from build123d import *

# Parameters (mm, degrees)
F0_R     = 14.2875
F1_DEPTH = 25.4
F2_DEPTH = 50.8


with BuildPart() as f1:
    # F0 (on Top) → F1 (new body)
    with BuildSketch(Plane.XY):
        with BuildLine():
            Line((9.780704698, 26.8489932886), (0, 28.575))
            ThreePointArc((0, 28.575), (-28.575, 0), (0, -28.575))
            Line((0, -28.575), (9.780704698, -26.8489932886))
            ThreePointArc((9.780704698, -26.8489932886), (23.4095521288, -16.3866864902), (28.575, 0))
            ThreePointArc((28.575, 0), (23.4095521288, 16.3866864902), (9.780704698, 26.8489932886))
        make_face()
        with BuildLine():
            ThreePointArc((-13.4703841816, 4.7625), (0, 14.2875), (13.4703841816, 4.7625))
            Line((13.4703841816, 4.7625), (19.05, 4.7625))
            Line((19.05, 4.7625), (19.05, -4.7625))
            Line((19.05, -4.7625), (13.4703841816, -4.7625))
            ThreePointArc((13.4703841816, -4.7625), (0, -14.2875), (-13.4703841816, -4.7625))
            Line((-13.4703841816, -4.7625), (-19.05, -4.7625))
            Line((-19.05, -4.7625), (-19.05, 4.7625))
            Line((-19.05, 4.7625), (-13.4703841816, 4.7625))
        make_face(mode=Mode.SUBTRACT)
        with BuildLine():
            ThreePointArc((9.780704698, 26.8489932886), (4.9659159165, 28.1401901932), (0, 28.575))
            Line((0, 28.575), (9.780704698, 26.8489932886))
        make_face()
        with BuildLine():
            Line((53.975, 19.05), (9.780704698, 26.8489932886))
            ThreePointArc((9.780704698, 26.8489932886), (23.4095521288, 16.3866864902), (28.575, 0))
            ThreePointArc((28.575, 0), (23.4095521288, -16.3866864902), (9.780704698, -26.8489932886))
            Line((9.780704698, -26.8489932886), (53.975, -19.05))
            ThreePointArc((53.975, -19.05), (34.925, 0), (53.975, 19.05))
        make_face()
        with BuildLine():
            ThreePointArc((73.025, 0), (67.4453841816, 13.4703841816), (53.975, 19.05))
            ThreePointArc((53.975, 19.05), (34.925, 0), (53.975, -19.05))
            ThreePointArc((53.975, -19.05), (67.4453841816, -13.4703841816), (73.025, 0))
        make_face()
        with Locations((53.975, 0)):
            Circle(F0_R, mode=Mode.SUBTRACT)
        with BuildLine():
            ThreePointArc((-13.4703841816, -4.7625), (-14.2875, 0), (-13.4703841816, 4.7625))
            Line((-13.4703841816, 4.7625), (-19.05, 4.7625))
            Line((-19.05, 4.7625), (-19.05, -4.7625))
            Line((-19.05, -4.7625), (-13.4703841816, -4.7625))
        make_face()
    extrude(amount=F1_DEPTH)

    # F0 (on Top) → F2 (join)
    with BuildSketch(Plane.XY):
        with BuildLine():
            ThreePointArc((9.780704698, 26.8489932886), (4.9659159165, 28.1401901932), (0, 28.575))
            Line((0, 28.575), (9.780704698, 26.8489932886))
        make_face()
        with BuildLine():
            Line((9.780704698, -26.8489932886), (0, -28.575))
            ThreePointArc((0, -28.575), (4.9659159165, -28.1401901932), (9.780704698, -26.8489932886))
        make_face()
        with BuildLine():
            Line((9.780704698, 26.8489932886), (0, 28.575))
            ThreePointArc((0, 28.575), (-28.575, 0), (0, -28.575))
            Line((0, -28.575), (9.780704698, -26.8489932886))
            ThreePointArc((9.780704698, -26.8489932886), (23.4095521288, -16.3866864902), (28.575, 0))
            ThreePointArc((28.575, 0), (23.4095521288, 16.3866864902), (9.780704698, 26.8489932886))
        make_face()
        with BuildLine():
            ThreePointArc((-13.4703841816, 4.7625), (0, 14.2875), (13.4703841816, 4.7625))
            Line((13.4703841816, 4.7625), (19.05, 4.7625))
            Line((19.05, 4.7625), (19.05, -4.7625))
            Line((19.05, -4.7625), (13.4703841816, -4.7625))
            ThreePointArc((13.4703841816, -4.7625), (0, -14.2875), (-13.4703841816, -4.7625))
            Line((-13.4703841816, -4.7625), (-19.05, -4.7625))
            Line((-19.05, -4.7625), (-19.05, 4.7625))
            Line((-19.05, 4.7625), (-13.4703841816, 4.7625))
        make_face(mode=Mode.SUBTRACT)
        with BuildLine():
            ThreePointArc((-13.4703841816, -4.7625), (-14.2875, 0), (-13.4703841816, 4.7625))
            Line((-13.4703841816, 4.7625), (-19.05, 4.7625))
            Line((-19.05, 4.7625), (-19.05, -4.7625))
            Line((-19.05, -4.7625), (-13.4703841816, -4.7625))
        make_face()
    extrude(amount=F2_DEPTH)


solid = f1.part
Geometry check sheet. Reference: the model listing, model coordinates, mm. A direction names the side the tool comes from. Round coordinates to 2 decimals unless told otherwise and drop trailing zeros. Write each loop counter-clockwise with the first axis right and the second up, starting at its lowest first coordinate (ties: lowest second). Pieces come first, ordered by that corner, then holes. Notation, with made-up numbers: (28, 63) -> (75, 63) arc R15 cw to (75, 68) -> close; hole circle Ø9 at (65, -28). An arc over 180 degrees is marked (long way). One line per item, written item: value. Start each with the question number.
(1) Cross-section at A-A, the plane x = 0. Record the cut outline in (y, z) (1 decimal), and give its area (3 significant figures).
(2) Go/stop test with flat-tipped pins: pin 1 Ø2 at (x, y) = (45.5, 12.5) entering from +Z; pin 2 Ø6 at (y, z) = (-2.5, 12) entering from -X (3 decimals); pin 3 Ø1.7 at (x, z) = (17, 17.5) entering from -Y (3 decimals); pin 4 Ø3 at (x, y) = (13, -8) entering from -Z. Record where each tip stops, or that it passes through.
(3) Cross-section at B-B, the plane z = 13. Give the number of separate pieces and of enclosed holes in the cut face, and give its area (3 significant figures).
(4) Access from +Z, -Z, +X, -X, +Y, -Y to the whole of each face (thin tool, end or side, straight path). Record for faces 4 (the cylindrical face through (-27.895, 6.194, 25.044)), 5 (the flat face through (22, 0, 0)), 6 (the flat face through (16, -4.762, 25)).
(5) Cross-section at D-D, the plane x = 66. Record the cut outline in (y, z).
(6) Draft check along Y on faces 1 (the flat face through (19.05, 0, 25)), 2 (the cylindrical face through (73.02, -0.42, 12.52)), 3 (the flat face through (31.6, -23, 12.5)). Enter one of: +Y half, -Y half, draft (parallel to the pull), parting line (faces both ways), or undercut.
(7) Scan lines: line 1 (X direction, y = -0.5, z = 38); line 2 (Z direction, x = 37, y = 16.5); line 3 (Y direction, x = -6, z = 34). Record each from-to range of solid material in increasing order. Write a range as [from, to].
Answer:
1. outline: (-28.6, 0) -> (-14.3, 0) -> (-14.3, 50.8) -> (-28.6, 50.8) -> close; (14.3, 0) -> (28.6, 0) -> (28.6, 50.8) -> (14.3, 50.8) -> close
1. area: 1,450 mm²
2. pin 1: z = 25.4
2. pin 2: x = -28.575
2. pin 3: y = -25.725
2. pin 4: z = 0
3. separate pieces: 1
3. enclosed holes: 2
3. area: 3,100 mm²
4. face 4: +Z
4. face 5: -Z, +X, -X, +Y, -Y
4. face 6: +Z, -Z
5. outline: (-14.78, 0) -> (-7.72, 0) -> (-7.72, 25.4) -> (-14.78, 25.4) -> close; (7.72, 0) -> (14.78, 0) -> (14.78, 25.4) -> (7.72, 25.4) -> close
6. face 1: undercut
6. face 2: parting line
6. face 3: -Y half
7. line 1: [-28.57, -14.28], [19.05, 28.57]
7. line 2: [0, 25.4]
7. line 3: [-27.94, -12.97], [12.97, 27.94]
